from build123d import *

# Parameters (mm, degrees)
SKETCH1_R           = 20
SKETCH1_W           = 65
SKETCH1_H           = 40
BOSS_EXTRUDE1_DEPTH = 6.35
SKETCH2_R           = 7.62
SKETCH2_R_2         = 2
CUT_EXTRUDE1_DEPTH  = 69.303166105
SKETCH4_W           = 15
SKETCH4_H           = 28
BOSS_EXTRUDE2_DEPTH = 10
CUT_EXTRUDE2_REACH  = 95.835
SKETCH5_W           = 15
SKETCH5_H           = 6.35
CUT_EXTRUDE3_REACH  = 78.19
SKETCH7_R           = 17.5
SKETCH7_R_2         = 13.5
CUT_EXTRUDE4_DEPTH  = 2
SKETCH8_R           = 2
BOSS_EXTRUDE3_DEPTH = 15


with BuildPart() as part:
    # Sketch1 → Boss-Extrude1 (new body)
    with BuildSketch(Plane.XY):
        Circle(SKETCH1_R)
        with Locations((32.5, 0)):
            Rectangle(SKETCH1_W, SKETCH1_H)
    extrude(amount=BOSS_EXTRUDE1_DEPTH)

    # Sketch2 → Cut-Extrude1 (cut, through all)
    with BuildSketch(Plane.XY.offset(6.35)):
        Circle(SKETCH2_R)
        with Locations((-1.350914013, 15.44101782)):
            Circle(SKETCH2_R_2)
        with Locations((12.696856686, 8.890434763)):
            Circle(SKETCH2_R_2)
        with Locations((14.047770699, -6.550583057)):
            Circle(SKETCH2_R_2)
        with Locations((1.350914013, -15.44101782)):
            Circle(SKETCH2_R_2)
        with Locations((-12.696856686, -8.890434763)):
            Circle(SKETCH2_R_2)
        with Locations((-14.047770699, 6.550583057)):
            Circle(SKETCH2_R_2)
    extrude(amount=-CUT_EXTRUDE1_DEPTH, mode=Mode.SUBTRACT)

    # Sketch4 → Boss-Extrude2 (add, symmetric)
    with BuildSketch(Plane(origin=(0, 0, 0), x_dir=(1, 0, 0), z_dir=(0, 1, 0))):
        with Locations((57.5, -20.35)):
            Rectangle(SKETCH4_W, SKETCH4_H)
    extrude(amount=BOSS_EXTRUDE2_DEPTH, both=True)

    # Sketch5 → Cut-Extrude2 (cut, up to next)
    with BuildSketch(Plane(origin=(65, 0, 0), x_dir=(0, 0, -1), z_dir=(1, 0, 0)), mode=Mode.PRIVATE) as cut_extrude2_sk1:
        with Locations((-26.85, 0)):
            Rectangle(SKETCH5_W, SKETCH5_H)
    cut_extrude2_tool1 = extrude(cut_extrude2_sk1.sketch, amount=-CUT_EXTRUDE2_REACH, mode=Mode.PRIVATE) & part.part
    add(cut_extrude2_tool1.solids().sort_by_distance((65, 0, 26.85))[0], mode=Mode.SUBTRACT)

    # Sketch6 → Cut-Extrude3 (cut, up to next)
    with BuildSketch(Plane(origin=(0, 0, 0), x_dir=(-1, 0, 0), z_dir=(0, 0, -1)), mode=Mode.PRIVATE) as cut_extrude3_sk1:
        with BuildLine():
            Line((-47.393320053, 2.55), (-44.046679947, 2.55))
            ThreePointArc((-44.046679947, 2.55), (-45.72, -3.05), (-47.393320053, 2.55))
        make_face()
    cut_extrude3_tool1 = extrude(cut_extrude3_sk1.sketch, amount=-CUT_EXTRUDE3_REACH, mode=Mode.PRIVATE) & part.part
    add(cut_extrude3_tool1.solids().sort_by_distance((45.72, -0.111199, 0))[0], mode=Mode.SUBTRACT)

    # Sketch7 → Cut-Extrude4 (cut)
    with BuildSketch(Plane(origin=(0, 0, 0), x_dir=(-1, 0, 0), z_dir=(0, 0, -1))):
        with Locations((-45.72, 0)):
            Circle(SKETCH7_R)
        with Locations((-45.72, 0)):
            Circle(SKETCH7_R_2, mode=Mode.SUBTRACT)
    extrude(amount=-CUT_EXTRUDE4_DEPTH, mode=Mode.SUBTRACT)

    # Sketch8 → Boss-Extrude3 (add)
    with BuildSketch(Plane(origin=(65, 0, 0), x_dir=(0, 0, -1), z_dir=(1, 0, 0))):
        with Locations((-31.35, 4.175)):
            Circle(SKETCH8_R)
    extrude(amount=-BOSS_EXTRUDE3_DEPTH)


solid = part.part
The listing builds one solid part. Answer for the finished solid, in the listing's coordinates (mm). A direction names the side the tool comes from. Coordinates: 2 decimals unless noted, no trailing zeros. Order: outer loops, then holes, each group sorted by start corner. A loop starts at its lowest first (then second) coordinate and runs counter-clockwise, first axis right, second up.
Q1. A cutting plane is placed at B-B, the plane x = 45.72. Write down the section's boundary in (y, z), and give its area (3 significant figures).
Q2. Consider line 1 (Y direction, x = 45.72, z = 3); line 2 (X direction, y = -7.5, z = 19.5); line 3 (Z direction, x = 5.5, y = -12). Determine where each line is inside the solid, lowest interval first.
Q3. A cutting plane is placed at C-C, the plane y = 0. Write down the section's boundary in (x, z).
Q4. Which of the six approach directions +Z, -Z, +X, -X, +Y, -Y give full straight-line access (tool end or side, diameter ignored) to faces 5 (the face through (57, 10, 20)), 6 (the face through (59.207, 0.594, 0.986)), 7 (the face through (50, 0, 17)), 8 (the face through (58, 3.175, 25)), 9 (the face through (57, -10, 20))?
Q5. Given P1, Ø4.5, axis at x = 54, z = 30.5, coming from the +Y side; P2, Ø1, axis at y = -0.5, z = 19, coming from the -X side; P3, Ø3.5, axis at x = 14.05, y = -6.55, coming from the -Z side; P4, Ø5, axis at x = 1.35, y = -15.44, coming from the +Z side, each flat-ended and moving along its own axis, determine where each tip first touches the part or whether it passes through.
Q6. For a pull along Z with two mould halves and no side action, classify faces 1 (the face through (57.605, 2.175, 31.379)), 2 (the face through (57, -7, 34.35)), 3 (the face through (12, 0, 0)), 4 (the face through (58, -3.175, 27)) as pulls with the +Z half, pulls with the -Z half, needs draft (parallel to the pull), parting line crosses it, or undercut.
Q7. A cutting plane is placed at A-A, the plane z = 26.5. Write down the section's boundary in (x, y) (3 decimals), and give its area (3 significant figures).
Q8. A cutting plane is placed at D-D, the plane z = 13. Write down the section's boundary in (x, y), and give its area (3 significant figures).
Answers follow:
1. outline: (-20, 0) - (-17.5, 0) - (-17.5, 2) - (-13.5, 2) - (-13.5, 0) - (-3.05, 0) - (-3.05, 6.35) - (-20, 6.35) - close; (2.55, 0) - (13.5, 0) - (13.5, 2) - (17.5, 2) - (17.5, 0) - (20, 0) - (20, 6.35) - (2.55, 6.35) - close
1. area: 202 mm2
2. line 1: y = -20 to -3.05, 2.55 to 20
2. line 2: x = 50 to 65
2. line 3: z = 0 to 6.35
3. outline: (-20, 0) - (-7.62, 0) - (-7.62, 6.35) - (-20, 6.35) - close; (7.62, 0) - (28.22, 0) - (28.22, 2) - (32.22, 2) - (32.22, 0) - (42.67, 0) - (42.67, 6.35) - (7.62, 6.35) - close; (48.77, 0) - (59.22, 0) - (59.22, 2) - (63.22, 2) - (63.22, 0) - (65, 0) - (65, 19.35) - (50, 19.35) - (50, 6.35) - (48.77, 6.35) - close
4. face 5: +Z, +X, -X, +Y
4. face 6: -Z
4. face 7: +Z, -X, +Y, -Y
4. face 8: +X, -X
4. face 9: +Z, +X, -X, -Y
5. P1: stops at y = 10
5. P2: stops at x = 50
5. P3: passes through
5. P4: stops at z = 6.35
6. face 1: undercut
6. face 2: pulls with the +Z half
6. face 3: pulls with the -Z half
6. face 4: needs draft
7. outline: (50, -10) - (65, -10) - (65, -3.175) - (50, -3.175) - close; (50, 3.175) - (65, 3.175) - (65, 10) - (50, 10) - close
7. area: 205 mm2
8. outline: (50, -10) - (65, -10) - (65, 10) - (50, 10) - close
8. area: 300 mm2
